Source: CAD feature listing. Evaluate the final solid. Frame: model axes, mm. A direction names the side the tool comes from. Give positions to 0.01 mm unless a question says otherwise; leave off trailing zeros. Loops run counter-clockwise (first coordinate to the right, second up) from the corner with the lowest first, then second, coordinate; pieces in that order, holes last. Notation, with made-up numbers: (77.5, -9) -> (99.5, -9) arc R12 cw to (99.5, -3) -> close; hole circle Ø11 at (-4.75, -11.75). An arc over 180 degrees is marked (long way). Put each result on its own line as item: value.
```python
from build123d import *

# Parameters (mm, degrees)
EXTRUDE_1_DEPTH     = 5
SKETCH_3_W          = 9
SKETCH_3_H          = 35.5
SKETCH_3_W_2        = 60
EXTRUDE_3_DEPTH     = 25
SKETCH_4_W          = 40
SKETCH_4_H          = 8
EXTRUDE_4_DEPTH     = 5
SKETCH_5_R          = 1.2
CUT_EXTRUDE_1_DEPTH = 210.737222495
SKETCH_6_W          = 40
SKETCH_6_H          = 8
EXTRUDE_5_DEPTH     = 5
EXTRUDE_6_DEPTH     = 2.5
SKETCH_8_W          = 40
SKETCH_8_H          = 8
EXTRUDE_7_DEPTH     = 5
SKETCH_17_W         = 40
SKETCH_17_H         = 8
EXTRUDE_12_DEPTH    = 5
SKETCH_18_W         = 25
SKETCH_18_H         = 25
CUT_EXTRUDE_3_DEPTH = 6
SKETCH_21_R         = 0.9
CUT_EXTRUDE_4_DEPTH = 10
SKETCH_22_R         = 1.2
CUT_EXTRUDE_5_DEPTH = 10
SKETCH_23_W         = 45
SKETCH_23_H         = 22
CUT_EXTRUDE_6_DEPTH = 5
SKETCH_25_R         = 1.3
CUT_EXTRUDE_7_DEPTH = 14
SKETCH_26_W         = 17.5
SKETCH_26_H         = 12
CUT_EXTRUDE_8_DEPTH = 15


with BuildPart() as part:
    # Sketch 1 → Extrude 1 (new body)
    with BuildSketch(Plane.XY):
        with BuildLine():
            Line((5, 0), (55, 0))
            ThreePointArc((55, 0), (58.535533906, -1.464466094), (60, -5))
            Line((60, -5), (60, -197.05))
            ThreePointArc((60, -197.05), (58.535533906, -200.585533906), (55, -202.05))
            Line((55, -202.05), (5, -202.05))
            ThreePointArc((5, -202.05), (1.464466094, -200.585533906), (0, -197.05))
            Line((0, -197.05), (0, -5))
            ThreePointArc((0, -5), (1.464466094, -1.464466094), (5, 0))
        make_face()
    extrude(amount=EXTRUDE_1_DEPTH)

    # Sketch 3 → Extrude 3 (add)
    with BuildSketch(Plane.XY.offset(5)):
        with Locations((-4.5, -22.75)):
            Rectangle(SKETCH_3_W, SKETCH_3_H)
        with Locations((30, -22.75)):
            Rectangle(SKETCH_3_W_2, SKETCH_3_H)
        with Locations((64.5, -22.75)):
            Rectangle(SKETCH_3_W, SKETCH_3_H)
        with Locations((-4.5, -179.3)):
            Rectangle(SKETCH_3_W, SKETCH_3_H)
        with Locations((30, -179.3)):
            Rectangle(SKETCH_3_W_2, SKETCH_3_H)
        with Locations((64.5, -179.3)):
            Rectangle(SKETCH_3_W, SKETCH_3_H)
    extrude(amount=-EXTRUDE_3_DEPTH)

    # Sketch 4 → Extrude 4 (add)
    with BuildSketch(Plane(origin=(0, -5, 0), x_dir=(1, 0, 0), z_dir=(0, 1, 0))):
        with Locations((30, 11)):
            Rectangle(SKETCH_4_W, SKETCH_4_H)
    extrude(amount=EXTRUDE_4_DEPTH)

    # Sketch 5 → Cut-Extrude 1 (cut, through all)
    with BuildSketch(Plane(origin=(0, -5, 0), x_dir=(1, 0, 0), z_dir=(0, 1, 0))):
        with Locations(Location((1, 15, 0), (0, 0, 270))):
            Circle(SKETCH_5_R)
        with Locations(Location((1, 5, 0), (0, 0, 270))):
            Circle(SKETCH_5_R)
        with Locations(Location((59, 5, 0), (0, 0, 270))):
            Circle(SKETCH_5_R)
        with Locations(Location((59, 15, 0), (0, 0, 270))):
            Circle(SKETCH_5_R)
    extrude(amount=-CUT_EXTRUDE_1_DEPTH, mode=Mode.SUBTRACT)

    # Sketch 6 → Extrude 5 (add)
    with BuildSketch(Plane.XZ.offset(197.05)):
        with Locations((30, -11)):
            Rectangle(SKETCH_6_W, SKETCH_6_H)
    extrude(amount=EXTRUDE_5_DEPTH)

    # Sketch 7 → Extrude 6 (add, symmetric)
    with BuildSketch(Plane(origin=(30, 0, 0), x_dir=(0, 0, -1), z_dir=(1, 0, 0))):
        with BuildLine():
            Line((20, -5), (30, -5))
            ThreePointArc((30, -5), (37.071067812, -7.928932188), (40, -15))
            Line((40, -15), (40, -187.05))
            ThreePointArc((40, -187.05), (37.071067812, -194.121067812), (30, -197.05))
            Line((30, -197.05), (20, -197.05))
            Line((20, -197.05), (20, -162.05))
            Line((20, -162.05), (25, -162.05))
            ThreePointArc((25, -162.05), (28.535533906, -160.585533906), (30, -157.05))
            Line((30, -157.05), (30, -45))
            ThreePointArc((30, -45), (28.535533906, -41.464466094), (25, -40))
            Line((25, -40), (20, -40))
            Line((20, -40), (20, -5))
        make_face()
    extrude(amount=EXTRUDE_6_DEPTH, both=True)

    # Sketch 8 → Extrude 7 (add)
    with BuildSketch(Plane(origin=(0, -161.55, 0), x_dir=(1, 0, 0), z_dir=(0, 1, 0))):
        with Locations((30, 11)):
            Rectangle(SKETCH_8_W, SKETCH_8_H)
    extrude(amount=EXTRUDE_7_DEPTH)

    # Sketch 17 → Extrude 12 (add)
    with BuildSketch(Plane.XZ.offset(40.5)):
        with Locations((30, -11)):
            Rectangle(SKETCH_17_W, SKETCH_17_H)
    extrude(amount=EXTRUDE_12_DEPTH)

    # Sketch 18 → Cut-Extrude 3 (cut)
    with BuildSketch(Plane.XY.offset(5)):
        with Locations((30, -179.55)):
            Rectangle(SKETCH_18_W, SKETCH_18_H)
    extrude(amount=-CUT_EXTRUDE_3_DEPTH, mode=Mode.SUBTRACT)

    # Sketch 21 → Cut-Extrude 4 (cut)
    with BuildSketch(Plane.XY.offset(5)):
        with Locations((20.5, -170.05)):
            Circle(SKETCH_21_R)
        with Locations((39.5, -170.05)):
            Circle(SKETCH_21_R)
        with Locations((39.5, -189.05)):
            Circle(SKETCH_21_R)
        with Locations((20.5, -189.05)):
            Circle(SKETCH_21_R)
        with BuildLine():
            Line((17.5, -187.05), (20.5, -187.05))
            ThreePointArc((20.5, -187.05), (21.914213562, -187.635786438), (22.5, -189.05))
            Line((22.5, -189.05), (22.5, -192.05))
            Line((22.5, -192.05), (37.5, -192.05))
            Line((37.5, -192.05), (37.5, -189.05))
            ThreePointArc((37.5, -189.05), (38.085786438, -187.635786438), (39.5, -187.05))
            Line((39.5, -187.05), (42.5, -187.05))
            Line((42.5, -187.05), (42.5, -172.05))
            Line((42.5, -172.05), (39.5, -172.05))
            ThreePointArc((39.5, -172.05), (38.085786438, -171.464213562), (37.5, -170.05))
            Line((37.5, -170.05), (37.5, -167.05))
            Line((37.5, -167.05), (22.5, -167.05))
            Line((22.5, -167.05), (22.5, -170.05))
            ThreePointArc((22.5, -170.05), (21.914213562, -171.464213562), (20.5, -172.05))
            Line((20.5, -172.05), (17.5, -172.05))
            Line((17.5, -172.05), (17.5, -187.05))
        make_face()
    extrude(amount=-CUT_EXTRUDE_4_DEPTH, mode=Mode.SUBTRACT)

    # Sketch 22 → Cut-Extrude 5 (cut)
    with BuildSketch(Plane.XY.offset(5)):
        with Locations((5.5, -140.55)):
            Circle(SKETCH_22_R)
        with Locations((54.5, -141.55)):
            Circle(SKETCH_22_R)
        with Locations((5.5, -72.55)):
            Circle(SKETCH_22_R)
        with Locations((54.5, -65.55)):
            Circle(SKETCH_22_R)
        with Locations((1, -22)):
            Circle(SKETCH_22_R)
        with Locations((59, -22)):
            Circle(SKETCH_22_R)
    extrude(amount=-CUT_EXTRUDE_5_DEPTH, mode=Mode.SUBTRACT)

    # Sketch 23 → Cut-Extrude 6 (cut)
    with BuildSketch(Plane.XY.offset(5)):
        with Locations((30, -22)):
            Rectangle(SKETCH_23_W, SKETCH_23_H)
    extrude(amount=-CUT_EXTRUDE_6_DEPTH, mode=Mode.SUBTRACT)

    # Sketch 25 → Cut-Extrude 7 (cut)
    with BuildSketch(Plane.XY):
        with Locations((45.5, -13.5)):
            Circle(SKETCH_25_R)
        with Locations((14.5, -30.5)):
            Circle(SKETCH_25_R)
        Polygon((52.5, -33), (52.5, -16), (42.5, -16), (42.5, -11), (7.5, -11), (7.5, -28), (17.5, -28), (17.5, -33), align=None)
    extrude(amount=-CUT_EXTRUDE_7_DEPTH, mode=Mode.SUBTRACT)

    # Sketch 26 → Cut-Extrude 8 (cut)
    with BuildSketch(Plane(origin=(0, 0, -20), x_dir=(-1, 0, 0), z_dir=(0, 0, -1))):
        with Locations((-41.25, -178.55)):
            Rectangle(SKETCH_26_W, SKETCH_26_H)
        with Locations((-41.25, -22)):
            Rectangle(SKETCH_26_W, SKETCH_26_H)
    cut_extrude_8 = extrude(amount=-CUT_EXTRUDE_8_DEPTH, mode=Mode.SUBTRACT)

    # Mirror 1: Cut-Extrude 8 across plane
    add(cut_extrude_8.mirror(Plane(origin=(30, 0, 0), x_dir=(0, 0, 1), z_dir=(1, 0, 0))), mode=Mode.SUBTRACT)


solid = part.part
```
(1) Section B-B on z = -22. Return loops of the section in (x, y), then the cut area to 3 significant figures.
Calculated:
outline: (27.5, -197.05) -> (32.5, -197.05) -> (32.5, -162.05) -> (27.5, -162.05) -> close; (27.5, -40) -> (32.5, -40) -> (32.5, -5) -> (27.5, -5) -> close
area: 350 mm²
(2) Line query: probe 1 along Y at (x, z) = (35.5, -18); probe 2 along X at (y, z) = (-189, -3); probe 3 along Y at (x, z) = (30.5, -3.5). Output: solid intervals per line, ascending. Write a range as from..to.
Calculated:
probe 1: y = -197.05..-184.55, -172.55..-161.55, -40.5..-28, -16..-5
probe 2: x = -9..19.6, 21.4..22.5, 37.5..38.6, 40.4..69
probe 3: y = -197.05..-192.05, -167.05..-161.55, -40.5..-33, -11..-5
(3) Section A-A on x = 63.5. Return loops of the section in (y, z), then the cut area to 4 significant figures.
Calculated:
outline: (-197.05, -20) -> (-161.55, -20) -> (-161.55, 5) -> (-197.05, 5) -> close; (-40.5, -20) -> (-5, -20) -> (-5, 5) -> (-40.5, 5) -> close
area: 1,775 mm²
(4) Reachability of faces 5 (the flat face through (29, -40.5, -5)), 6 (the flat face through (46, -178, -5)), 7 (the flat face through (42.5, -14, -7)) from +Z, -Z, +X, -X, +Y, -Y: full face, straight path, thin tool, end or side. Return the list, or none.
Calculated:
face 5: none
face 6: -Z
face 7: +Z
(5) Draft query along X for faces 1 (the flat face through (-9, -180, -7)), 2 (the flat face through (30, -200, -7)), 3 (the flat face through (69, -180, -7)), 4 (the flat face through (14, -178, -5)). Return one class per face: released by +X, released by -X, zero draft, split by the parting line, or undercut.
Calculated:
face 1: released by -X
face 2: zero draft
face 3: released by +X
face 4: undercut
(6) First-contact query: P1, Ø4, axis at y = -2, z = -12.5, coming from the -X side; P2, Ø3, axis at x = 56, y = -114, coming from the -Z side; P3, Ø4, axis at x = 45.5, y = -13.5, coming from the +Z side. Flat tips, straight axial feed; report the tip coordinate or a pass-through.
Calculated:
P1: stops at x = 10
P2: stops at z = 0
P3: stops at z = 0
